Could you check a few things on this drawing? It's one solid part, dimensions in mm from its lowest x, y, z. A direction names the side the tool comes from. Round coordinates to 2 decimals unless told otherwise and drop trailing zeros. Loops run counter-clockwise (first coordinate to the right, second up) from the corner with the lowest first, then second, coordinate; pieces in that order, holes last. Notation, with made-up numbers: (-20.5, 23) -> (35.5, 23) arc R18 cw to (35.5, 54) -> close; hole circle Ø9 at (79.25, -0.5). An arc over 180 degrees is marked (long way). Put each result on its own line as item: value. Start each with the question number.
1. I need wall thicknesses on line 1 (X direction, y = 78.75, z = 7.5); line 2 (Y direction, x = 149.5, z = 7.5); line 3 (Y direction, x = 108, z = 8). Which ranges of each line are inside material? Lowest first, please. Write a range as [from, to].
2. Which directions (+Z, -Z, +X, -X, +Y, -Y) give clear straight access to the entire face, cutting with the end or side of a thin tool? Please do the marked faces 1 and 2.
3. Imagine slicing it at B-B, the plane z = 13.5. Please give me the cut outline in (x, y), and give its area (3 significant figures).
4. Imagine slicing it at A-A, the plane x = 48. Please give me the cut outline in (y, z).
5. Imagine slicing it at D-D, the plane y = 32.5. Please give me the cut outline in (x, z).
6. Imagine slicing it at C-C, the plane x = 16.5. Please give me the cut outline in (y, z).
7. I'm going to push flat-ended pins straight in: P1, Ø6, axis at y = 17.5, z = 7.5, coming from the -X side; P2, Ø6, axis at x = 28, z = 7.5, coming from the +Y side; P3, Ø5.5, axis at y = 67.5, z = 7.5, coming from the +X side; P4, Ø4.5, axis at x = 128, z = 7.5, coming from the +Y side. Where does each tip first touch, or does it pass through?
8. If we mould it in two halves opening along Y, with no side actions, what happens to the marked faces 3, 4 and 5? For each: pulls with the +Y half, pulls with the -Y half, needs draft (parallel to the pull), parting line crosses it, or undercut.
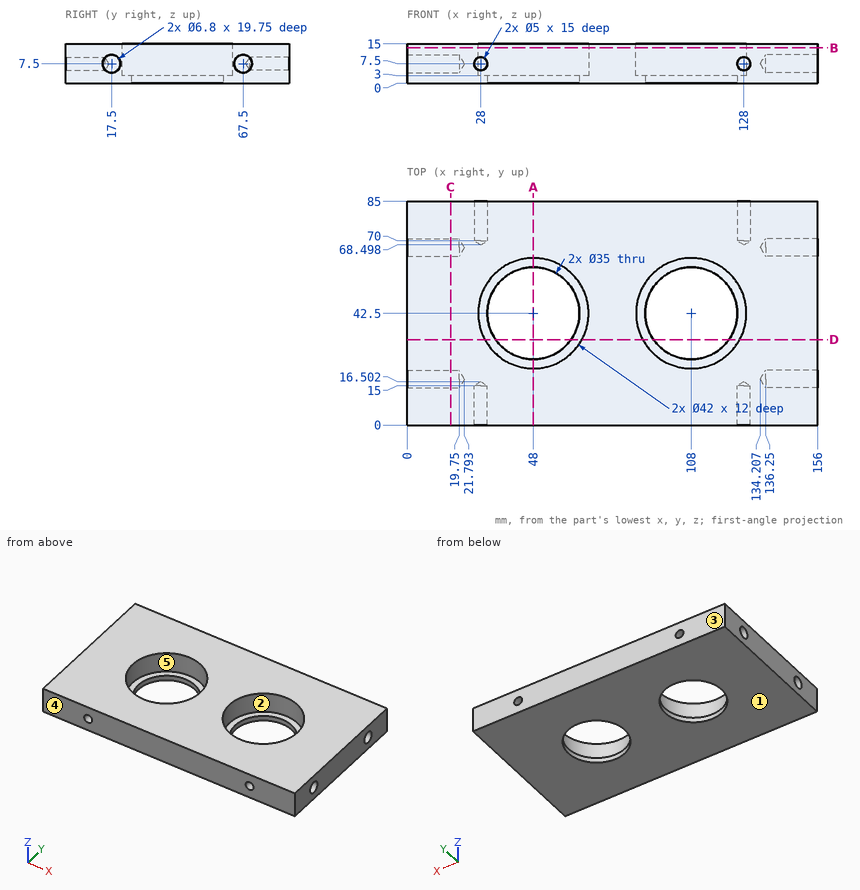
Entries:
1. line 1: [0, 25.5], [30.5, 125.5], [130.5, 156]
1. line 2: [0, 14.1], [20.9, 64.1], [70.9, 85]
1. line 3: [0, 21.5], [63.5, 85]
2. face 1: -Z, +X, -X, +Y, -Y
2. face 2: +Z
3. outline: (0, 0) -> (156, 0) -> (156, 85) -> (0, 85) -> close; hole circle Ø42 at (48, 42.5); hole circle Ø42 at (108, 42.5)
3. area: 10,500 mm^2
4. outline: (0, 0) -> (25, 0) -> (25, 3) -> (21.5, 3) -> (21.5, 15) -> (0, 15) -> close; (60, 0) -> (85, 0) -> (85, 15) -> (63.5, 15) -> (63.5, 3) -> (60, 3) -> close
5. outline: (0, 0) -> (33.64, 0) -> (33.64, 3) -> (29.53, 3) -> (29.53, 15) -> (0, 15) -> close; (62.36, 0) -> (93.64, 0) -> (93.64, 3) -> (89.53, 3) -> (89.53, 15) -> (66.47, 15) -> (66.47, 3) -> (62.36, 3) -> close; (122.36, 0) -> (156, 0) -> (156, 15) -> (126.47, 15) -> (126.47, 3) -> (122.36, 3) -> close
6. outline: (0, 0) -> (85, 0) -> (85, 15) -> (0, 15) -> close; hole circle Ø6.8 at (17.5, 7.5); hole circle Ø6.8 at (67.5, 7.5)
7. P1: x = 19.99
7. P2: y = 85
7. P3: x = 135.86
7. P4: y = 69.85
8. face 3: pulls with the +Y half
8. face 4: pulls with the -Y half
8. face 5: undercut
